```python
from build123d import *

# Parameters (mm, degrees)
SKETCH1_W           = 96.27
SKETCH1_H           = 112
BOSS_EXTRUDE1_DEPTH = 73.8
SKETCH2_W           = 86.27
SKETCH2_H           = 102
CUT_EXTRUDE1_DEPTH  = 68.8
FILLET1_R           = 10
FILLET2_R           = 10
FILLET3_R           = 7.5
FILLET4_R           = 7.5
FILLET6_R           = 5
SKETCH3_R           = 3.04
CUT_EXTRUDE2_DEPTH  = 5
SKETCH4_R           = 10.75
CUT_EXTRUDE3_DEPTH  = 5
SKETCH5_R           = 2.5
CUT_EXTRUDE4_DEPTH  = 5
HOLE1_START         = 43.135
HOLE1_OUTLINE_R     = 1.4224
HOLE1_DEPTH         = 5


# Read off the part's stored shape, not the designer's step: Hole1
# Some blends are built 0.0001 mm under size
with BuildPart() as part:
    # Sketch1 → Boss-Extrude1 (new body)
    with BuildSketch(Plane(origin=(0, 0, 0), x_dir=(1, 0, 0), z_dir=(0, 1, 0))):
        Rectangle(SKETCH1_W, SKETCH1_H)
    extrude(amount=BOSS_EXTRUDE1_DEPTH)

    # Sketch2 → Cut-Extrude1 (cut)
    with BuildSketch(Plane.XZ):
        Rectangle(SKETCH2_W, SKETCH2_H)
    extrude(amount=-CUT_EXTRUDE1_DEPTH, mode=Mode.SUBTRACT)

    # Fillet1
    fillet1_edges = [part.edges().sort_by_distance(p)[0] for p in [
        (-48.135, 73.8, 0),
        (0, 73.8, 56),
        (48.135, 73.8, 0),
        (0, 73.8, -56),
    ]]
    fillet(fillet1_edges, radius=FILLET1_R)

    # Fillet2
    # the kernel refuses this fillet: 10 mm, written as the material it takes off along each edge
    with BuildSketch(Plane(origin=(38.135, 63.8, 46), x_dir=(1, 0, 0), z_dir=(0, 0, 1))) as fillet2_piece_1_section:
        Polygon((0, 0), (FILLET2_R, 0), (FILLET2_R, FILLET2_R), (0, FILLET2_R), align=None)
    fillet2_piece_1 = extrude(amount=FILLET2_R, mode=Mode.PRIVATE)
    fillet2_piece_1 = fillet2_piece_1 - Plane(origin=(38.135, 63.8, 46), x_dir=(-0.7071067811865475, -0.7071067811865475, 0), z_dir=(0, 0, 1)) * Sphere(FILLET2_R, mode=Mode.PRIVATE)
    add(fillet2_piece_1, mode=Mode.SUBTRACT)
    with BuildSketch(Plane(origin=(-38.135, 63.8, 46), x_dir=(-1, 0, 0), z_dir=(0, 0, 1))) as fillet2_piece_2_section:
        Polygon((0, 0), (FILLET2_R, 0), (FILLET2_R, -FILLET2_R), (0, -FILLET2_R), align=None)
    fillet2_piece_2 = extrude(amount=FILLET2_R, mode=Mode.PRIVATE)
    fillet2_piece_2 = fillet2_piece_2 - Plane(origin=(-38.135, 63.8, 46), x_dir=(0.7071067811865475, -0.7071067811865475, 0), z_dir=(0, 0, 1)) * Sphere(FILLET2_R, mode=Mode.PRIVATE)
    add(fillet2_piece_2, mode=Mode.SUBTRACT)
    with BuildSketch(Plane(origin=(38.135, 63.8, -46), x_dir=(0, 0, -1), z_dir=(1, 0, 0))) as fillet2_piece_3_section:
        Polygon((0, 0), (FILLET2_R, 0), (FILLET2_R, FILLET2_R), (0, FILLET2_R), align=None)
    fillet2_piece_3 = extrude(amount=FILLET2_R, mode=Mode.PRIVATE)
    fillet2_piece_3 = fillet2_piece_3 - Plane(origin=(38.135, 63.8, -46), x_dir=(0, -0.7071067811865475, 0.7071067811865475), z_dir=(1, 0, 0)) * Sphere(FILLET2_R, mode=Mode.PRIVATE)
    add(fillet2_piece_3, mode=Mode.SUBTRACT)
    with BuildSketch(Plane(origin=(-38.135, 63.8, -46), x_dir=(0, 0, -1), z_dir=(-1, 0, 0))) as fillet2_piece_4_section:
        Polygon((0, 0), (FILLET2_R, 0), (FILLET2_R, -FILLET2_R), (0, -FILLET2_R), align=None)
    fillet2_piece_4 = extrude(amount=FILLET2_R, mode=Mode.PRIVATE)
    fillet2_piece_4 = fillet2_piece_4 - Plane(origin=(-38.135, 63.8, -46), x_dir=(0, -0.7071067811865475, 0.7071067811865475), z_dir=(-1, 0, 0)) * Sphere(FILLET2_R, mode=Mode.PRIVATE)
    add(fillet2_piece_4, mode=Mode.SUBTRACT)
    with BuildSketch(Plane(origin=(-48.135, -25, -56), x_dir=(0, 0, 1), z_dir=(0, 1, 0)), Plane(origin=(-48.135, -25, 56), x_dir=(1, 0, 0), z_dir=(0, 1, 0))) as fillet2_piece_5:
        with BuildLine():
            CenterArc((FILLET2_R, FILLET2_R), FILLET2_R, 180, 90)
            Line((0, FILLET2_R), (0, 0))
            Line((0, 0), (FILLET2_R, 0))
        make_face()
    extrude(amount=88.8, mode=Mode.SUBTRACT)
    with BuildSketch(Plane(origin=(48.135, -25, -56), x_dir=(0, 0, 1), z_dir=(0, 1, 0)), Plane(origin=(48.135, -25, 56), x_dir=(-1, 0, 0), z_dir=(0, 1, 0))) as fillet2_piece_6:
        with BuildLine():
            CenterArc((FILLET2_R, -FILLET2_R), FILLET2_R, 90, 90)
            Line((0, -FILLET2_R), (0, 0))
            Line((0, 0), (FILLET2_R, 0))
        make_face()
    extrude(amount=88.8, mode=Mode.SUBTRACT)

    # Fillet3
    fillet3_edges = [part.edges().sort_by_distance(p)[0] for p in [
        (43.135, 68.8, 0),
        (0, 68.8, -51),
        (-43.135, 68.8, 0),
        (0, 68.8, 51),
    ]]
    fillet(fillet3_edges, radius=FILLET3_R)

    # Fillet4
    # the kernel refuses this fillet: 7.5 mm, written as the material it adds along each edge
    with BuildSketch(Plane(origin=(-35.635, 61.3, -43.5), x_dir=(0, 0, -1), z_dir=(-1, 0, 0))) as fillet4_piece_1_section:
        Polygon((0, 0), (FILLET4_R, 0), (FILLET4_R, -FILLET4_R), (0, -FILLET4_R), align=None)
    fillet4_piece_1 = extrude(amount=FILLET4_R, mode=Mode.PRIVATE)
    fillet4_piece_1 = fillet4_piece_1 - Plane(origin=(-35.635, 61.3, -43.5), x_dir=(0, -0.7071067811865475, 0.7071067811865475), z_dir=(-1, 0, 0)) * Sphere(FILLET4_R, mode=Mode.PRIVATE)
    add(fillet4_piece_1)
    with BuildSketch(Plane(origin=(-35.635, 61.3, 43.5), x_dir=(0, 0, 1), z_dir=(-1, 0, 0))) as fillet4_piece_2_section:
        Polygon((0, 0), (FILLET4_R, 0), (FILLET4_R, FILLET4_R), (0, FILLET4_R), align=None)
    fillet4_piece_2 = extrude(amount=FILLET4_R, mode=Mode.PRIVATE)
    fillet4_piece_2 = fillet4_piece_2 - Plane(origin=(-35.635, 61.3, 43.5), x_dir=(0, -0.7071067811865475, -0.7071067811865475), z_dir=(-1, 0, 0)) * Sphere(FILLET4_R, mode=Mode.PRIVATE)
    add(fillet4_piece_2)
    with BuildSketch(Plane(origin=(35.635, 61.3, -43.5), x_dir=(1, 0, 0), z_dir=(0, 0, -1))) as fillet4_piece_3_section:
        Polygon((0, 0), (FILLET4_R, 0), (FILLET4_R, -FILLET4_R), (0, -FILLET4_R), align=None)
    fillet4_piece_3 = extrude(amount=FILLET4_R, mode=Mode.PRIVATE)
    fillet4_piece_3 = fillet4_piece_3 - Plane(origin=(35.635, 61.3, -43.5), x_dir=(-0.7071067811865475, -0.7071067811865475, 0), z_dir=(0, 0, -1)) * Sphere(FILLET4_R, mode=Mode.PRIVATE)
    add(fillet4_piece_3)
    with BuildSketch(Plane(origin=(35.635, 61.3, 43.5), x_dir=(1, 0, 0), z_dir=(0, 0, 1))) as fillet4_piece_4_section:
        Polygon((0, 0), (FILLET4_R, 0), (FILLET4_R, FILLET4_R), (0, FILLET4_R), align=None)
    fillet4_piece_4 = extrude(amount=FILLET4_R, mode=Mode.PRIVATE)
    fillet4_piece_4 = fillet4_piece_4 - Plane(origin=(35.635, 61.3, 43.5), x_dir=(-0.7071067811865475, -0.7071067811865475, 0), z_dir=(0, 0, 1)) * Sphere(FILLET4_R, mode=Mode.PRIVATE)
    add(fillet4_piece_4)
    with BuildSketch(Plane(origin=(43.135, 0, 51), x_dir=(-1, 0, 0), z_dir=(0, 1, 0)), Plane(origin=(-43.135, 0, 51), x_dir=(0, 0, -1), z_dir=(0, 1, 0))) as fillet4_piece_5:
        with BuildLine():
            CenterArc((FILLET4_R, -FILLET4_R), FILLET4_R, 90, 90)
            Line((0, -FILLET4_R), (0, 0))
            Line((0, 0), (FILLET4_R, 0))
        make_face()
    extrude(amount=61.3)
    with BuildSketch(Plane(origin=(43.135, 0, -51), x_dir=(-1, 0, 0), z_dir=(0, 1, 0)), Plane(origin=(-43.135, 0, -51), x_dir=(0, 0, 1), z_dir=(0, 1, 0))) as fillet4_piece_6:
        with BuildLine():
            CenterArc((FILLET4_R, FILLET4_R), FILLET4_R, 180, 90)
            Line((0, FILLET4_R), (0, 0))
            Line((0, 0), (FILLET4_R, 0))
        make_face()
    extrude(amount=61.3)

    # Fillet6
    fillet6_edges = [part.edges().sort_by_distance(p)[0] for p in [
        (-48.135, 0, 0),
        (48.135, 0, 0),
        (0, 0, 56),
        (0, 0, -56),
        (-45.206067812, 0, 53.071067812),
        (45.206067812, 0, 53.071067812),
        (45.206067812, 0, -53.071067812),
        (-45.206067812, 0, -53.071067812),
    ]]
    fillet(fillet6_edges, radius=FILLET6_R - 0.0001)  # a hair under: the kernel refuses the full size

    # Sketch3 → Cut-Extrude2 (cut)
    with BuildSketch(Plane(origin=(0, 73.8, 0), x_dir=(1, 0, 0), z_dir=(0, 1, 0))):
        with Locations(Location((19.265, -11, 0), (0, 0, 270))):
            Circle(SKETCH3_R)
        with Locations(Location((11.765, -11, 0), (0, 0, 270))):
            Circle(SKETCH3_R)
    extrude(amount=-CUT_EXTRUDE2_DEPTH, mode=Mode.SUBTRACT)

    # Sketch4 → Cut-Extrude3 (cut)
    with BuildSketch(Plane(origin=(0, 73.8, 0), x_dir=(1, 0, 0), z_dir=(0, 1, 0))):
        with Locations(Location((-18.135, -26, 0), (0, 0, 270))):
            Circle(SKETCH4_R)
    extrude(amount=-CUT_EXTRUDE3_DEPTH, mode=Mode.SUBTRACT)

    # Sketch5 → Cut-Extrude4 (cut)
    with BuildSketch(Plane(origin=(0, 73.8, 0), x_dir=(1, 0, 0), z_dir=(0, 1, 0))):
        with Locations(Location((9.865, -20.3, 0), (0, 0, 270))):
            Circle(SKETCH5_R)
        with Locations(Location((17.865, -20.3, 0), (0, 0, 270))):
            Circle(SKETCH5_R)
    extrude(amount=-CUT_EXTRUDE4_DEPTH, mode=Mode.SUBTRACT)

    # Hole1 outline → Hole1 (cut)
    with BuildSketch(Plane.YZ.offset(HOLE1_START)):
        with Locations((53.8, 0)):
            Circle(HOLE1_OUTLINE_R)
    extrude(amount=HOLE1_DEPTH, mode=Mode.SUBTRACT)


solid = part.part
```
Read the model definition and answer for the solid it produces. Units are mm, in the model's axes. A direction names the side the tool comes from. Round coordinates to 2 decimals unless told otherwise and drop trailing zeros. Write each loop counter-clockwise with the first axis right and the second up, starting at its lowest first coordinate (ties: lowest second). Pieces come first, ordered by that corner, then holes. Notation, with made-up numbers: (47, 51.5) -> (56, 51.5) arc R28 ccw to (56, 75.5) -> close; hole circle Ø3 at (41, -19). An arc over 180 degrees is marked (long way). Answer in a Markdown table with one row per item. Add a question column.
1) Given P1, Ø8, axis at x = -19.5, z = -33, coming from the -Y side; P2, Ø5.5, axis at x = 19.265, z = 11, coming from the +Y side; P3, Ø1.5, axis at y = 66, z = 26, coming from the -X side; P4, Ø2.5, axis at y = 53.8, z = 0, coming from the +X side (3 decimals), each flat-ended and moving along its own axis, determine where each tip first touches the part or whether it passes through.
2) Determine the mould class of faces 1 (the face through (-46.631, 1.426, -0.644)), 2 (the face through (45.283, 33.988, -52.993)), 3 (the face through (43.135, 30, -1)) for opening direction X: pulls with the +X half, pulls with the -X half, needs draft (parallel to the pull), parting line crosses it, or undercut.
3) Find section A-A, the plane z = 11. State how many separate pieces and enclosed holes the cut face has, and give its area (3 significant figures).
4) Find section B-B, the plane y = 57.5. Determine the outline of the cut face in (x, z) (3 decimals).
5) Consider line 1 (Z direction, x = -13.5, y = 11); line 2 (X direction, y = 70.8, z = 20.3) (3 decimals); line 3 (X direction, y = 53, z = -5) (3 decimals). Determine where each line is inside the solid, lowest interval first.
6) Which of the six approach directions +Z, -Z, +X, -X, +Y, -Y give full straight-line access (tool end or side, diameter ignored) to faces 4 (the face through (0, 30, -51)), 5 (the face through (45.6, 55.114, -0.545)), 6 (the face through (13.82, 71.33, 8.76))?
Findings below:
| question | item | result |
|---|---|---|
| 1 | P1 | y = 68.8 |
| 1 | P2 | through |
| 1 | P3 | x = -48.03 |
| 1 | P4 | x = -43.135 |
| 2 | face 1 | pulls with the -X half |
| 2 | face 2 | pulls with the +X half |
| 2 | face 3 | undercut |
| 3 | separate pieces | 3 |
| 3 | enclosed holes | 0 |
| 3 | area | 1,080 mm² |
| 4 | outline | (-48.135, -46) arc R10 ccw to (-38.135, -56) -> (38.135, -56) arc R10 ccw to (48.135, -46) -> (48.135, 46) arc R10 ccw to (38.135, 56) -> (-38.135, 56) arc R10 ccw to (-48.135, 46) -> close; hole (-43.135, -43.5) arc R7.5 ccw to (-35.635, -51) -> (35.635, -51) arc R7.5 ccw to (43.135, -43.5) -> (43.135, 43.5) arc R7.5 ccw to (35.635, 51) -> (-35.635, 51) arc R7.5 ccw to (-43.135, 43.5) -> close |
| 5 | line 1 | -56 to -51, 51 to 56 |
| 5 | line 2 | -45.276 to -27.249, -9.021 to 7.365, 12.365 to 15.365, 20.365 to 45.276 |
| 5 | line 3 | -48.135 to -43.135, 43.135 to 48.135 |
| 6 | face 4 | -Y |
| 6 | face 5 | +X |
| 6 | face 6 | +Y, -Y |
